Read the model definition and answer for the solid it produces. Units are mm, in the model's axes. A direction names the side the tool comes from. Give positions to 0.01 mm unless a question says otherwise; leave off trailing zeros. Write each loop counter-clockwise with the first axis right and the second up, starting at its lowest first coordinate (ties: lowest second). Pieces come first, ordered by that corner, then holes.
```python
from build123d import *

# Parameters (mm, degrees)
SKETCH_R                = 2.1
POCKET_DEPTH            = 5
SKETCH002_R             = 2.1
POCKET001_DEPTH         = 7
BODY001_ROLL_ANGLE      = 90
BODY001_PLACEMENT_ANGLE = 90


with BuildPart() as part:
    # Sketch001 → Revolution001 (revolve)
    with BuildSketch(Plane.XY):
        Polygon((28, 0), (32, 11.6), (32, 51), (14, 51), (14, 53), (0, 53), (0, 0), (0, -30), (5, -30), (5, 0), align=None)
    revolve(axis=Axis((0, 0, 0), (0, 1, 0)))

    # Sketch → Pocket (cut)
    with BuildSketch(Plane.XZ):
        with Locations((-15.556349, 15.556349)):
            Circle(SKETCH_R)
        with Locations((15.556349, 15.556349)):
            Circle(SKETCH_R)
        with Locations((15.556349, -15.556349)):
            Circle(SKETCH_R)
        with Locations((-15.556349, -15.556349)):
            Circle(SKETCH_R)
    extrude(amount=-POCKET_DEPTH, mode=Mode.SUBTRACT)

    # Sketch002 (on Face16 of Pocket) → Pocket001 (cut)
    with BuildSketch(Plane(origin=(0, 53, 0), x_dir=(-1, 0, 0), z_dir=(0, 1, 0))):
        with Locations((-11, 0)):
            Circle(SKETCH002_R)
        with Locations((0, -11)):
            Circle(SKETCH002_R)
        with Locations((11, 0)):
            Circle(SKETCH002_R)
        with Locations((0, 11)):
            Circle(SKETCH002_R)
    extrude(amount=-POCKET001_DEPTH, mode=Mode.SUBTRACT)


with BuildPart() as part_1:
    # Body001 roll: moved
    add(part.part.rotate(Axis((0, 0, 0), (1, 0, 0)), BODY001_ROLL_ANGLE))


with BuildPart() as part_2:
    # Body001 placement: moved
    add(part_1.part.moved(Location((0, 0, -36.75))).rotate(Axis((0, 0, -36.75), (0, 0, 1)), BODY001_PLACEMENT_ANGLE))


solid = part_2.part
```
Item 1: Section A-A (x = 0) is taken. Write down the section's boundary in (y, z), and give its area (3 significant figures).
Result set:
outline: (-32, -25.15) - (-28, -36.75) - (-5, -36.75) - (-5, -66.75) - (5, -66.75) - (5, -36.75) - (28, -36.75) - (32, -25.15) - (32, 14.25) - (14, 14.25) - (14, 16.25) - (13.1, 16.25) - (13.1, 9.25) - (8.9, 9.25) - (8.9, 16.25) - (-8.9, 16.25) - (-8.9, 9.25) - (-13.1, 9.25) - (-13.1, 16.25) - (-14, 16.25) - (-14, 14.25) - (-32, 14.25) - close
area: 3,510 mm2
Item 2: Each of these flat-tipped pins is pushed along its axis until it touches: pin 1 Ø1.5 at (x, y) = (14.5, 11) entering from +Z; pin 2 Ø2 at (x, y) = (-15.5, -16) entering from -Z; pin 3 Ø3.5 at (x, y) = (-10.5, 0) entering from +Z; pin 4 Ø8 at (y, z) = (15, -6.5) entering from +X. Where does it stop, or does it pass through?
Result set:
pin 1: stops at z = 14.25
pin 2: stops at z = -31.75
pin 3: stops at z = 16.25
pin 4: stops at x = 30.05
Item 3: Section C-C (z = -8.5) is taken. Write down the section's boundary in (x, y), and give its area (3 significant figures).
Result set:
outline: circle Ø64 at (0, 0)
area: 3,220 mm2
Item 4: Which of the six approach directions +Z, -Z, +X, -X, +Y, -Y give full straight-line access (tool end or side, diameter ignored) to faces 1 (the flat face through (0, 0, -66.75)), 2 (the cylindrical face through (-8.918, 0.273, 12.799)), 3 (the flat face through (16, 16, -31.75))?
Result set:
face 1: -Z, +X, -X, +Y, -Y
face 2: +Z
face 3: -Z
Item 5: Determine the mould class of faces 4 (the flat face through (7, 14, 14.25)), 5 (the flat face through (16, -16, -31.75)), 6 (the cylindrical face through (3, -4, -52)) for opening direction Y: pulls with the +Y half, pulls with the -Y half, needs draft (parallel to the pull), parting line crosses it, or undercut.
Result set:
face 4: needs draft
face 5: undercut
face 6: parting line crosses it
Item 6: Find the intervals of material crossed by line 1 along Z through (x, y) = (10, 23); line 2 along Y through (x, z) = (-27.5, -24.5); line 3 along X through (y, z) = (-2.5, 4.5), in increasing order.
Result set:
line 1: z = -36.75 to 14.25
line 2: y = -16.36 to 16.36
line 3: x = -31.9 to 31.9
Item 7: Section B-B (z = -44.5) is taken. Write down the section's boundary in (x, y), and give its area (3 significant figures).
Result set:
outline: circle Ø10 at (0, 0)
area: 78.5 mm2
